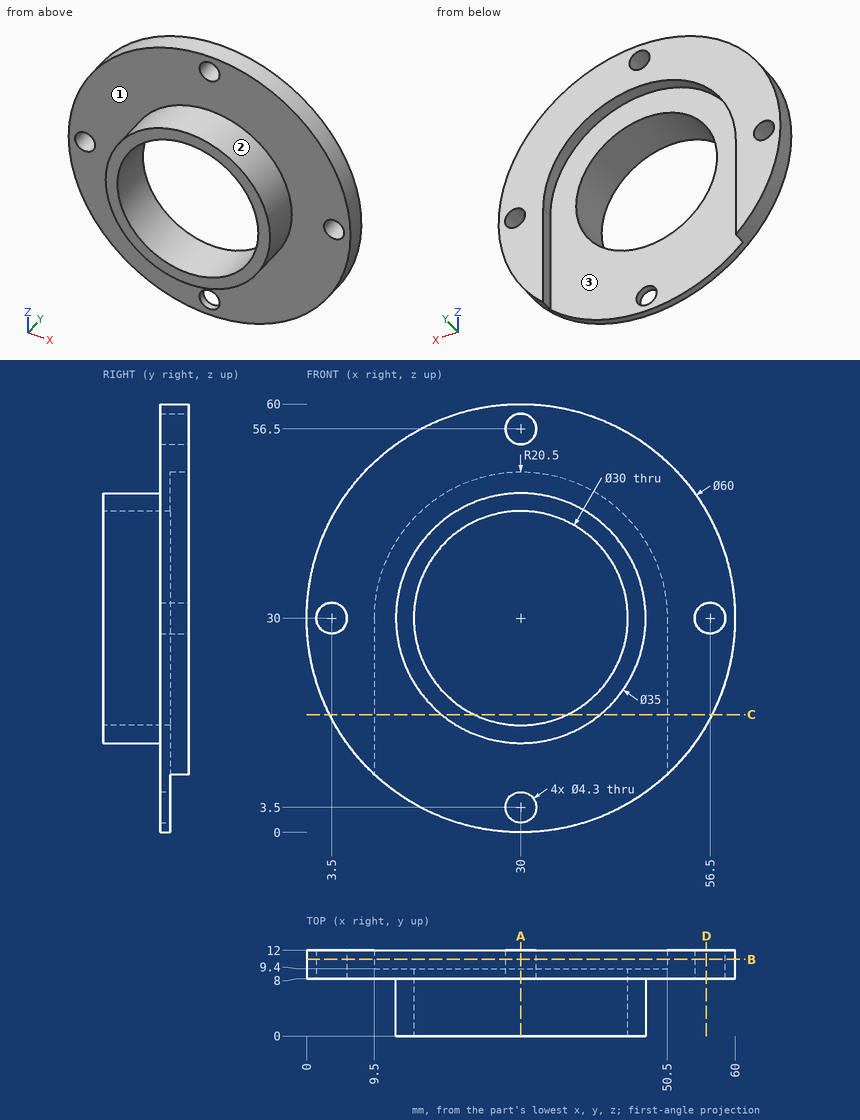
Source: three-view drawing plus pictorial views. Frame: mm from the lowest corner of the part. Round coordinates to 2 decimals unless told otherwise and drop trailing zeros. Loops run counter-clockwise (first coordinate to the right, second up) from the corner with the lowest first, then second, coordinate; pieces in that order, holes last.
Q1. Section D-D on x = 56. Return loops of the section in (y, z), plus the area to 3 significant figures.
Q2. Pull-direction query (X, two-part tool) for the marked faces 1, 2 and 3; classes: released by +X, released by -X, zero draft, split by the parting line, or undercut.
Q3. Pin query (flat end, axial travel): P1, Ø0.8, axis at y = 11, z = 24, coming from the +X side; P2, Ø5.5, axis at x = 56.5, z = 30, coming from the -Y side; P3, Ø1.5, axis at y = 8.5, z = 23.5, coming from the +X side. Return the tip coordinate at first contact, or that it passes through.
Q4. Section C-C on z = 16.5. Return loops of the section in (x, y), plus the area to 3 significant figures.
Q5. Section A-A on x = 30. Return loops of the section in (y, z).
Q6. Material intervals for L1, parallel to Z at x = 30, y = 9; L2, parallel to X at y = 11.1, z = 30; L3, parallel to Z at x = 30, y = 3.25, sorted ascending.
Q7. Section B-B on y = 10.75. Return loops of the section in (x, z), plus the area to 3 significant figures.
Evaluation:
1. outline: (8, 15.03) - (12, 15.03) - (12, 27.91) - (8, 27.91) - close; (8, 32.09) - (12, 32.09) - (12, 44.97) - (8, 44.97) - close
1. area: 103 mm2
2. face 1: zero draft
2. face 2: split by the parting line
2. face 3: undercut
3. P1: stops at x = 59.47
3. P2: stops at y = 8
3. P3: stops at x = 59.44
4. outline: (3.21, 8) - (18.86, 8) - (18.86, 0) - (23.46, 0) - (23.46, 9.4) - (9.5, 9.4) - (9.5, 12) - (3.21, 12) - close; (36.54, 0) - (41.14, 0) - (41.14, 8) - (56.79, 8) - (56.79, 12) - (50.5, 12) - (50.5, 9.4) - (36.54, 9.4) - close
4. area: 163 mm2
5. outline: (0, 12.5) - (8, 12.5) - (8, 5.65) - (9.4, 5.65) - (9.4, 15) - (0, 15) - close; (0, 45) - (9.4, 45) - (9.4, 50.5) - (12, 50.5) - (12, 54.35) - (8, 54.35) - (8, 47.5) - (0, 47.5) - close; (8, 0) - (9.4, 0) - (9.4, 1.35) - (8, 1.35) - close; (8, 58.65) - (12, 58.65) - (12, 60) - (8, 60) - close
6. L1: z = 0 to 1.35, 5.65 to 15, 45 to 54.35, 58.65 to 60
6. L2: x = 0 to 1.35, 5.65 to 9.5, 50.5 to 54.35, 58.65 to 60
6. L3: z = 12.5 to 15, 45 to 47.5
7. outline: (9.5, 8.1) - (9.5, 30) arc R20.5 cw to (50.5, 30) - (50.5, 8.1) arc R30 ccw (long way) to start; hole circle Ø4.3 at (3.5, 30); hole circle Ø4.3 at (30, 56.5); hole circle Ø4.3 at (56.5, 30)
7. area: 998 mm2
